The listing builds one solid part. Answer for the finished solid, in the listing's coordinates (mm). Face numbers are marked on the shaded views. A direction names the side the tool comes from. Coordinates: 2 decimals unless noted, no trailing zeros. Loops run counter-clockwise (first coordinate to the right, second up) from the corner with the lowest first, then second, coordinate; pieces in that order, holes last. Notation, with made-up numbers: M 20.25,8.25 L 77.25,8.25 A5 cw 77.25,17.25 Z; hole C 34,70.25 d5. An arc over 180 degrees is marked long. Return JSON: item names as keys, results as strings. Group by question number.
1. Straight lines are drawn through the part: L1, parallel to Y at x = 14, z = 12; L2, parallel to Y at x = 73, z = 12; L3, parallel to Y at x = 66, z = 43. For each, find the intervals that lie inside material, in ascending order. Write a range as from..to.
2. Section C-C (x = 75) is taken. Write down the section's boundary in (y, z).
3. Section A-A (z = 34) is taken. Write down the section's boundary in (x, y), then the cut area to 3 significant figures.
4. Section B-B (y = -18) is taken. Write down the section's boundary in (x, z).
5. Section D-D (y = -45) is taken. Write down the section's boundary in (x, z).
6. Which of the six approach directions +Z, -Z, +X, -X, +Y, -Y give full straight-line access (tool end or side, diameter ignored) to the marked faces 1, 2 and 3?
7. Given P1, Ø1.5, axis at x = 16, z = 39, coming from the -Y side; P2, Ø3.5, axis at x = 10, z = 33.5, coming from the +Y side; P3, Ø12.5, axis at x = 14, y = -18, coming from the -Z side, each flat-ended and moving along its own axis, determine where each tip first touches the part or whether it passes through.
```python
from build123d import *

# Parameters (mm, degrees)
SKETCH1_R           = 7
BOSS_EXTRUDE1_DEPTH = 45
CHAMFER1_SIZE       = 7
CHAMFER2_SIZE       = 7
CHAMFER3_SIZE       = 5
FILLET1_R           = 5


with BuildPart() as part:
    # Sketch1 → Boss-Extrude1 (new body)
    with BuildSketch(Plane.XY):
        with BuildLine():
            Line((14, 0), (0, 0))
            Line((0, 0), (0, -32))
            Line((0, -32), (42.863608631, -32))
            ThreePointArc((42.863608631, -32), (44.694157304, -42.140064899), (49.954706191, -51))
            Line((49.954706191, -51), (57.451644827, -51))
            Line((57.451644827, -51), (84, -16))
            Line((84, -16), (84, 8))
            Line((84, 8), (55, 8))
            ThreePointArc((55, 8), (46.591637328, -1.464097542), (34.104042352, -3.544885088))
            Line((34.104042352, -3.544885088), (14, 0))
        make_face()
        with Locations((14, -18)):
            Circle(SKETCH1_R, mode=Mode.SUBTRACT)
    extrude(amount=BOSS_EXTRUDE1_DEPTH)

    # Chamfer1
    chamfer1_edges = [part.edges().sort_by_distance(p)[0] for p in [
        (0, 0, 22.5),
    ]]
    chamfer(chamfer1_edges, length=CHAMFER1_SIZE)

    # Chamfer2
    chamfer2_edges = [part.edges().sort_by_distance(p)[0] for p in [
        (0, -32, 22.5),
    ]]
    chamfer(chamfer2_edges, length=CHAMFER2_SIZE)

    # Chamfer3
    chamfer3_edges = [part.edges().sort_by_distance(p)[0] for p in [
        (84, 8, 22.5),
    ]]
    chamfer(chamfer3_edges, length=CHAMFER3_SIZE)

    # Fillet1
    fillet1_edges = [part.edges().sort_by_distance(p)[0] for p in [
        (42.863608631, -32, 22.5),
    ]]
    fillet(fillet1_edges, radius=FILLET1_R)


solid = part.part
```
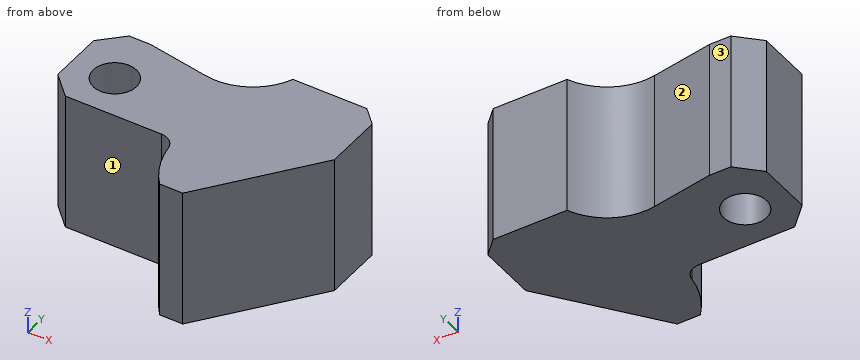
Worked out:
{
 "1": {"L1": "-32..-25, -11..0", "L2": "-30.5..8", "L3": "-39.73..8"},
 "2": {"outline": "M -27.87,0 L 8,0 L 8,45 L -27.87,45 Z"},
 "3": {"outline": "M 0,-25 L 7,-32 L 38.23,-32 A5 cw 43.18,-36.26 A29 ccw 49.95,-51 L 57.45,-51 L 84,-16 L 84,3 L 79,8 L 55,8 A19 cw 34.1,-3.54 L 14,0 L 7,0 L 0,-7 Z; hole C 14,-18 d14", "area": "2,930 mm^2"},
 "4": {"outline": "M 0,0 L 7,0 L 7,45 L 0,45 Z; M 21,0 L 82.48,0 L 82.48,45 L 21,45 Z"},
 "5": {"outline": "M 45.94,0 L 62,0 L 62,45 L 45.94,45 Z"},
 "6": {"face 1": "+Z, -Z, -X, -Y", "face 2": "+Z, -Z, +Y", "face 3": "+Z, -Z, -X, +Y"},
 "7": {"P1": "y = -32", "P2": "y = 0", "P3": "through"}
}
